from build123d import *

# Parameters (mm, degrees)
SKETCH_R  = 4.19854
PAD_DEPTH = 5


with BuildPart() as part:
    # Sketch → Pad (new body)
    with BuildSketch(Plane.XZ):
        with BuildLine():
            Line((-74.76046, 53.421562), (-74.76046, 105.632532))
            ThreePointArc((-74.76046, 105.632532), (-113.884518, 96.986251), (-147.92625, 75.853087))
            ThreePointArc((-191.195978, 51.976961), (-168.240252, 61.521279), (-147.92625, 75.853087))
            ThreePointArc((-191.195978, 51.976961), (-232.525307, -12.219718), (-208.043261, -84.538155))
            Line((-108.653475, -84.538155), (-208.043261, -84.538155))
            ThreePointArc((-108.653475, -84.538155), (-97.779522, -78.707083), (-96.619688, -66.422986))
            ThreePointArc((-76.988182, 47.66843), (-103.469883, -6.509598), (-96.619688, -66.422986))
            ThreePointArc((-76.988182, 47.66843), (-75.336834, 50.336871), (-74.76046, 53.421562))
        make_face()
        with Locations((-108.43, -63.28574)):
            Circle(SKETCH_R, mode=Mode.SUBTRACT)
        with Locations((-87.308784, 53.70005)):
            Circle(SKETCH_R, mode=Mode.SUBTRACT)
        with BuildLine():
            ThreePointArc((-129.83, 56.8), (-153.326605, -6.587909), (-128.84, -69.6))
            ThreePointArc((-128.84, -69.6), (-119.974424, -69.628015), (-117.608236, -61.08399))
            ThreePointArc((-104.620375, 37.907127), (-122.131275, -10.14298), (-117.608236, -61.08399))
            ThreePointArc((-104.620375, 37.907127), (-108.458862, 59.050873), (-129.83, 56.8))
        make_face(mode=Mode.SUBTRACT)
    extrude(amount=PAD_DEPTH)


solid = part.part
Read the model definition and answer for the solid it produces. Units are mm, in the model's axes. A direction names the side the tool comes from. Give positions to 0.01 mm unless a question says otherwise; leave off trailing zeros. Loops run counter-clockwise (first coordinate to the right, second up) from the corner with the lowest first, then second, coordinate; pieces in that order, holes last. Notation, with made-up numbers: (43.5, -9) -> (102.5, -9) arc R11 ccw to (102.5, 3) -> close; hole circle Ø2 at (-13.5, 72.5). An arc over 180 degrees is marked (long way). Use a Markdown table: item, result.
Q1. Determine the mould class of faces 1 (the face through (-153.33, -2.46, -5.62)), 2 (the face through (-74.76, -2, 79)), 3 (the face through (-155, 0, -9)), 4 (the face through (-168.55, -2.46, 61.35)) for opening direction X: pulls with the +X half, pulls with the -X half, needs draft (parallel to the pull), parting line crosses it, or undercut.
Solved:
| item | result |
|---|---|
| face 1 | undercut |
| face 2 | pulls with the +X half |
| face 3 | needs draft |
| face 4 | pulls with the -X half |
Q2. A tool of negligible diameter and unlimited length cuts with its end or side. For faces 5 (the face through (-122.035, -2.465, -9.428)), 6 (the face through (-158, -2, -84.538)), from which of +Z, -Z, +X, -X, +Y, -Y can it reach the whole face along a straight path? Write none if from no direction.
Solved:
| item | result |
|---|---|
| face 5 | +Y, -Y |
| face 6 | -Z, +X, -X, +Y, -Y |
Q3. Section A-A, the plane z = -15 is taken. Determine the outline of the cut face in (x, y), then the cut area to 3 significant figures.
Solved:
| item | result |
|---|---|
| outline | (-232.82, -5) -> (-152.89, -5) -> (-152.89, 0) -> (-232.82, 0) -> close; (-122.67, -5) -> (-104.58, -5) -> (-104.58, 0) -> (-122.67, 0) -> close |
| area | 490 mm^2 |
Q4. Section B-B, the plane y = -2.95 is taken. Determine the outline of the cut face in (x, z), then the cut area to 3 significant figures.
Solved:
| item | result |
|---|---|
| outline | (-208.04, -84.54) -> (-108.65, -84.54) arc R13.05 ccw to (-96.62, -66.42) arc R107.52 cw to (-76.99, 47.67) arc R8.54 ccw to (-74.76, 53.42) -> (-74.76, 105.63) arc R119.08 ccw to (-147.93, 75.85) arc R113.03 cw to (-191.2, 51.98) arc R87.91 ccw to start; hole (-129.83, 56.8) arc R95.24 ccw to (-128.84, -69.6) arc R7.31 ccw to (-117.61, -61.08) arc R117.69 cw to (-104.62, 37.91) arc R15.8 ccw to start; hole circle Ø8.4 at (-108.43, -63.29); hole circle Ø8.4 at (-87.31, 53.7) |
| area | 16,800 mm^2 |
Q5. Section D-D, the plane x = -100 is taken. Determine the outline of the cut face in (y, z).
Solved:
| item | result |
|---|---|
| outline | (-5, -81.26) -> (0, -81.26) -> (0, -57.24) -> (-5, -57.24) -> close; (-5, 7.75) -> (0, 7.75) -> (0, 101.66) -> (-5, 101.66) -> close |
Q6. Section C-C, the plane x = -120 is taken. Determine the outline of the cut face in (y, z), then the cut area to 3 significant figures.
Solved:
| item | result |
|---|---|
| outline | (-5, -84.54) -> (0, -84.54) -> (0, -69.65) -> (-5, -69.65) -> close; (-5, -52.42) -> (0, -52.42) -> (0, 1.51) -> (-5, 1.51) -> close; (-5, 62.07) -> (0, 62.07) -> (0, 94.29) -> (-5, 94.29) -> close |
| area | 505 mm^2 |
Q7. Find the intervals of material crossed by line 1 along Z through (x, y) = (-106, -2.6); line 2 along Z through (x, y) = (-108.43, -2.35); line 3 along X through (y, z) = (-3.25, 56), in increasing order.
Solved:
| item | result |
|---|---|
| line 1 | z = -84.27 to -66.71, -59.86 to 35.69, 56.76 to 99.88 |
| line 2 | z = -84.54 to -67.48, -59.09 to 31.51, 59.03 to 99.05 |
| line 3 | x = -179.74 to -130.52, -105.38 to -90.82, -83.8 to -74.76 |
Q8. This flat-tipped pin is pushed along its axis until it touches: pin 1 (9.5 mm diameter, centred on x = -108.43, z = -63.29, fed in from +Y). Where does it stop, or does it pass through?
Solved:
| item | result |
|---|---|
| pin 1 | stops at y = 0 |
